Could you check a few things on this model? Use its own coordinates, in mm. A direction names the side the tool comes from. Coordinates: 2 decimals unless noted, no trailing zeros. Loops run counter-clockwise (first coordinate to the right, second up) from the corner with the lowest first, then second, coordinate; pieces in that order, holes last.
from build123d import *

# Parameters (mm, degrees)
SKETCH_1_R          = 28.3
EXTRUDE_1_DEPTH     = 2
SKETCH_2_R          = 5
SKETCH_2_R_2        = 2
SKETCH_2_R_3        = 1.3
CUT_EXTRUDE_1_DEPTH = 41.072184867
CUT_EXTRUDE_3_DEPTH = 40.315613947
FILLET_2_R          = 2
FILLET_1_R          = 1


with BuildPart() as part:
    # ｽｹｯﾁ1 → ﾎﾞｽ - 押し出し1 (new body)
    with BuildSketch(Plane.XY):
        Circle(SKETCH_1_R)
    extrude(amount=EXTRUDE_1_DEPTH)

    # ｽｹｯﾁ2 → ｶｯﾄ - 押し出し1 (cut, through all)
    with BuildSketch(Plane.XY.offset(2)):
        Circle(SKETCH_2_R)
        with Locations((8.660254038, 5)):
            Circle(SKETCH_2_R_2)
        with Locations((8.660254038, -5)):
            Circle(SKETCH_2_R_2)
        with Locations((0, -10)):
            Circle(SKETCH_2_R_2)
        with Locations((-8.660254038, -5)):
            Circle(SKETCH_2_R_2)
        with Locations((-8.660254038, 5)):
            Circle(SKETCH_2_R_2)
        with Locations((0, 10)):
            Circle(SKETCH_2_R_2)
        with Locations((11.25, 19.485571585)):
            Circle(SKETCH_2_R_3)
        with Locations((22.5, 0)):
            Circle(SKETCH_2_R_3)
        with Locations((11.25, -19.485571585)):
            Circle(SKETCH_2_R_3)
        with Locations((-11.25, -19.485571585)):
            Circle(SKETCH_2_R_3)
        with Locations((-22.5, 0)):
            Circle(SKETCH_2_R_3)
        with Locations((-11.25, 19.485571585)):
            Circle(SKETCH_2_R_3)
        with BuildLine():
            Line((7.75, 24.325), (10, 24.325))
            Line((10, 24.325), (10, 22.275))
            Line((10, 22.275), (7.75, 22.275))
            Line((7.75, 22.275), (7.75, 15.8))
            Line((7.75, 15.8), (-7.75, 15.8))
            Line((-7.75, 15.8), (-7.75, 22.275))
            Line((-7.75, 22.275), (-10, 22.275))
            Line((-10, 22.275), (-10, 24.325))
            Line((-10, 24.325), (-7.75, 24.325))
            Line((-7.75, 24.325), (-7.75, 27.21814652))
            ThreePointArc((-7.75, 27.21814652), (0, 28.3), (7.75, 27.21814652))
            Line((7.75, 27.21814652), (7.75, 24.325))
        make_face()
        with BuildLine():
            Line((24.941067947, 5.450803121), (26.066067947, 3.502245962))
            Line((26.066067947, 3.502245962), (24.290715869, 2.477245962))
            Line((24.290715869, 2.477245962), (23.165715869, 4.425803121))
            Line((23.165715869, 4.425803121), (17.55820138, 1.188303121))
            Line((17.55820138, 1.188303121), (9.80820138, 14.611696879))
            Line((9.80820138, 14.611696879), (15.415715869, 17.849196879))
            Line((15.415715869, 17.849196879), (14.290715869, 19.797754038))
            Line((14.290715869, 19.797754038), (16.066067947, 20.822754038))
            Line((16.066067947, 20.822754038), (17.191067947, 18.874196879))
            Line((17.191067947, 18.874196879), (19.69660633, 20.320770139))
            ThreePointArc((19.69660633, 20.320770139), (24.508518927, 14.15), (27.44660633, 6.897376381))
            Line((27.44660633, 6.897376381), (24.941067947, 5.450803121))
        make_face()
        with BuildLine():
            Line((17.191067947, -18.874196879), (16.066067947, -20.822754038))
            Line((16.066067947, -20.822754038), (14.290715869, -19.797754038))
            Line((14.290715869, -19.797754038), (15.415715869, -17.849196879))
            Line((15.415715869, -17.849196879), (9.80820138, -14.611696879))
            Line((9.80820138, -14.611696879), (17.55820138, -1.188303121))
            Line((17.55820138, -1.188303121), (23.165715869, -4.425803121))
            Line((23.165715869, -4.425803121), (24.290715869, -2.477245962))
            Line((24.290715869, -2.477245962), (26.066067947, -3.502245962))
            Line((26.066067947, -3.502245962), (24.941067947, -5.450803121))
            Line((24.941067947, -5.450803121), (27.44660633, -6.897376381))
            ThreePointArc((27.44660633, -6.897376381), (24.508518927, -14.15), (19.69660633, -20.320770139))
            Line((19.69660633, -20.320770139), (17.191067947, -18.874196879))
        make_face()
        with BuildLine():
            Line((-7.75, -24.325), (-10, -24.325))
            Line((-10, -24.325), (-10, -22.275))
            Line((-10, -22.275), (-7.75, -22.275))
            Line((-7.75, -22.275), (-7.75, -15.8))
            Line((-7.75, -15.8), (7.75, -15.8))
            Line((7.75, -15.8), (7.75, -22.275))
            Line((7.75, -22.275), (10, -22.275))
            Line((10, -22.275), (10, -24.325))
            Line((10, -24.325), (7.75, -24.325))
            Line((7.75, -24.325), (7.75, -27.21814652))
            ThreePointArc((7.75, -27.21814652), (0, -28.3), (-7.75, -27.21814652))
            Line((-7.75, -27.21814652), (-7.75, -24.325))
        make_face()
        with BuildLine():
            Line((-24.941067947, -5.450803121), (-26.066067947, -3.502245962))
            Line((-26.066067947, -3.502245962), (-24.290715869, -2.477245962))
            Line((-24.290715869, -2.477245962), (-23.165715869, -4.425803121))
            Line((-23.165715869, -4.425803121), (-17.55820138, -1.188303121))
            Line((-17.55820138, -1.188303121), (-9.80820138, -14.611696879))
            Line((-9.80820138, -14.611696879), (-15.415715869, -17.849196879))
            Line((-15.415715869, -17.849196879), (-14.290715869, -19.797754038))
            Line((-14.290715869, -19.797754038), (-16.066067947, -20.822754038))
            Line((-16.066067947, -20.822754038), (-17.191067947, -18.874196879))
            Line((-17.191067947, -18.874196879), (-19.69660633, -20.320770139))
            ThreePointArc((-19.69660633, -20.320770139), (-24.508518927, -14.15), (-27.44660633, -6.897376381))
            Line((-27.44660633, -6.897376381), (-24.941067947, -5.450803121))
        make_face()
        with BuildLine():
            Line((-17.191067947, 18.874196879), (-16.066067947, 20.822754038))
            Line((-16.066067947, 20.822754038), (-14.290715869, 19.797754038))
            Line((-14.290715869, 19.797754038), (-15.415715869, 17.849196879))
            Line((-15.415715869, 17.849196879), (-9.80820138, 14.611696879))
            Line((-9.80820138, 14.611696879), (-17.55820138, 1.188303121))
            Line((-17.55820138, 1.188303121), (-23.165715869, 4.425803121))
            Line((-23.165715869, 4.425803121), (-24.290715869, 2.477245962))
            Line((-24.290715869, 2.477245962), (-26.066067947, 3.502245962))
            Line((-26.066067947, 3.502245962), (-24.941067947, 5.450803121))
            Line((-24.941067947, 5.450803121), (-27.44660633, 6.897376381))
            ThreePointArc((-27.44660633, 6.897376381), (-24.508518927, 14.15), (-19.69660633, 20.320770139))
            Line((-19.69660633, 20.320770139), (-17.191067947, 18.874196879))
        make_face()
    extrude(amount=-CUT_EXTRUDE_1_DEPTH, mode=Mode.SUBTRACT)

    # ｽｹｯﾁ3 → ｶｯﾄ - 押し出し3 (cut, through all)
    with BuildSketch(Plane.XY.offset(2)):
        with BuildLine():
            ThreePointArc((7.75, 27.21814652), (13.394592318, 23.200114441), (19.69660633, 20.320770139))
            ThreePointArc((19.69660633, 20.320770139), (14.15, 24.508518927), (7.75, 27.21814652))
        make_face()
        with BuildLine():
            ThreePointArc((27.44660633, 6.897376381), (26.789184636, 0), (27.44660633, -6.897376381))
            ThreePointArc((27.44660633, -6.897376381), (28.3, 0), (27.44660633, 6.897376381))
        make_face()
        with BuildLine():
            ThreePointArc((19.69660633, -20.320770139), (13.394592318, -23.200114441), (7.75, -27.21814652))
            ThreePointArc((7.75, -27.21814652), (14.15, -24.508518927), (19.69660633, -20.320770139))
        make_face()
        with BuildLine():
            ThreePointArc((-7.75, -27.21814652), (-13.394592318, -23.200114441), (-19.69660633, -20.320770139))
            ThreePointArc((-19.69660633, -20.320770139), (-14.15, -24.508518927), (-7.75, -27.21814652))
        make_face()
        with BuildLine():
            ThreePointArc((-27.44660633, -6.897376381), (-26.789184636, 0), (-27.44660633, 6.897376381))
            ThreePointArc((-27.44660633, 6.897376381), (-28.3, 0), (-27.44660633, -6.897376381))
        make_face()
        with BuildLine():
            ThreePointArc((-19.69660633, 20.320770139), (-13.394592318, 23.200114441), (-7.75, 27.21814652))
            ThreePointArc((-7.75, 27.21814652), (-14.15, 24.508518927), (-19.69660633, 20.320770139))
        make_face()
    extrude(amount=-CUT_EXTRUDE_3_DEPTH, mode=Mode.SUBTRACT)

    # ﾌｨﾚｯﾄ2
    fillet_2_edges = [part.edges().sort_by_distance(p)[0] for p in [
        (9.80820138, -14.611696879, 1),
        (17.55820138, -1.188303121, 1),
        (17.55820138, 1.188303121, 1),
        (9.80820138, 14.611696879, 1),
        (7.75, 15.8, 1),
        (-7.75, 15.8, 1),
        (-9.80820138, 14.611696879, 1),
        (-17.55820138, 1.188303121, 1),
        (-7.75, -15.8, 1),
        (7.75, -15.8, 1),
        (-17.55820138, -1.188303121, 1),
        (-9.80820138, -14.611696879, 1),
    ]]
    fillet(fillet_2_edges, radius=FILLET_2_R)

    # ﾌｨﾚｯﾄ1
    fillet_1_edges = [part.edges().sort_by_distance(p)[0] for p in [
        (27.44660633, -6.897376381, 1),
        (19.69660633, -20.320770139, 1),
        (19.69660633, 20.320770139, 1),
        (27.44660633, 6.897376381, 1),
        (-7.75, 27.21814652, 1),
        (7.75, 27.21814652, 1),
        (-27.44660633, 6.897376381, 1),
        (-19.69660633, 20.320770139, 1),
        (7.75, -27.21814652, 1),
        (-7.75, -27.21814652, 1),
        (-19.69660633, -20.320770139, 1),
        (-27.44660633, -6.897376381, 1),
    ]]
    fillet(fillet_1_edges, radius=FILLET_1_R)


solid = part.part
(1) I need wall thicknesses on probe 1 along Y at (x, z) = (0, 1.65); probe 2 along Y at (x, z) = (-17, 0.35); probe 3 along Y at (x, z) = (-12, 0.35). Which ranges of each line are inside material? Lowest first, please.
Answers:
probe 1: y = -15.8 to -12, -8 to -5, 5 to 8, 12 to 15.8
probe 2: y = -21.38 to -19.21, -2.39 to 2.39, 19.21 to 21.38
probe 3: y = -24.05 to -20.55, -18.42 to -15.88, -10.82 to 10.82, 15.88 to 18.42, 20.55 to 24.05
(2) Imagine slicing it at B-B, the plane y = 0. Write out the boundary of the cut face in (x, z).
Answers:
outline: (-26.79, 0) - (-23.8, 0) - (-23.8, 2) - (-26.79, 2) - close; (-21.2, 0) - (-5, 0) - (-5, 2) - (-21.2, 2) - close; (5, 0) - (21.2, 0) - (21.2, 2) - (5, 2) - close; (23.8, 0) - (26.79, 0) - (26.79, 2) - (23.8, 2) - close
(3) Which directions (+Z, -Z, +X, -X, +Y, -Y) give clear straight access to the entire face, cutting with the end or side of a thin tool? Please do faces 5 (the face through (0, -15.8, 1)), 6 (the face through (13.451, 16.715, 1.014)), 7 (the face through (25.2, 3, 1)).
Answers:
face 5: +Z, -Z, -Y
face 6: +Z, -Z, +X
face 7: +Z, -Z
(4) Imagine slicing it at C-C, the plane y = 10. Write out the boundary of the cut face in (x, z).
Answers:
outline: (-12.47, 0) - (-2, 0) - (-2, 2) - (-12.47, 2) - close; (2, 0) - (12.47, 0) - (12.47, 2) - (2, 2) - close
(5) Imagine slicing it at D-D, the plane x = -22.5. Write out the boundary of the cut face in (y, z).
Answers:
outline: (-4.04, 0) - (-1.3, 0) - (-1.3, 2) - (-4.04, 2) - close; (1.3, 0) - (4.04, 0) - (4.04, 2) - (1.3, 2) - close
(6) We'd pull the mould along X, two halves only. Please class faces 1 (the face through (13.51, -16.75, 1.01)), 2 (the face through (-13.643, 7.97, 1.014)), 3 (the face through (-10.614, -14.418, 0.986)), 4 (the face through (7.75, -20, 1)): +X half, -X half, draft (parallel to the pull), parting line (faces both ways), or undercut.
Answers:
face 1: +X half
face 2: undercut
face 3: -X half
face 4: undercut
(7) For pin 1 (1 mm diameter, centred on x = -0.5, z = 1, fed in from +Y); pin 2 (0.6 mm diameter, centred on y = 23.5, z = 1, fed in from -X); pin 3 (1 mm diameter, centred on y = -20, z = 1, fed in from +X), each with a flat end and sliding along its axis, tell me the tip position at first contact or that it passes through.
Answers:
pin 1: stops at y = 15.8
pin 2: stops at x = -13.39
pin 3: stops at x = 18.37
(8) Imagine slicing it at A-A, the plane x = 0. Write out the boundary of the cut face in (y, z), and give its area (3 significant figures).
Answers:
outline: (-15.8, 0) - (-12, 0) - (-12, 2) - (-15.8, 2) - close; (-8, 0) - (-5, 0) - (-5, 2) - (-8, 2) - close; (5, 0) - (8, 0) - (8, 2) - (5, 2) - close; (12, 0) - (15.8, 0) - (15.8, 2) - (12, 2) - close
area: 27.2 mm2
